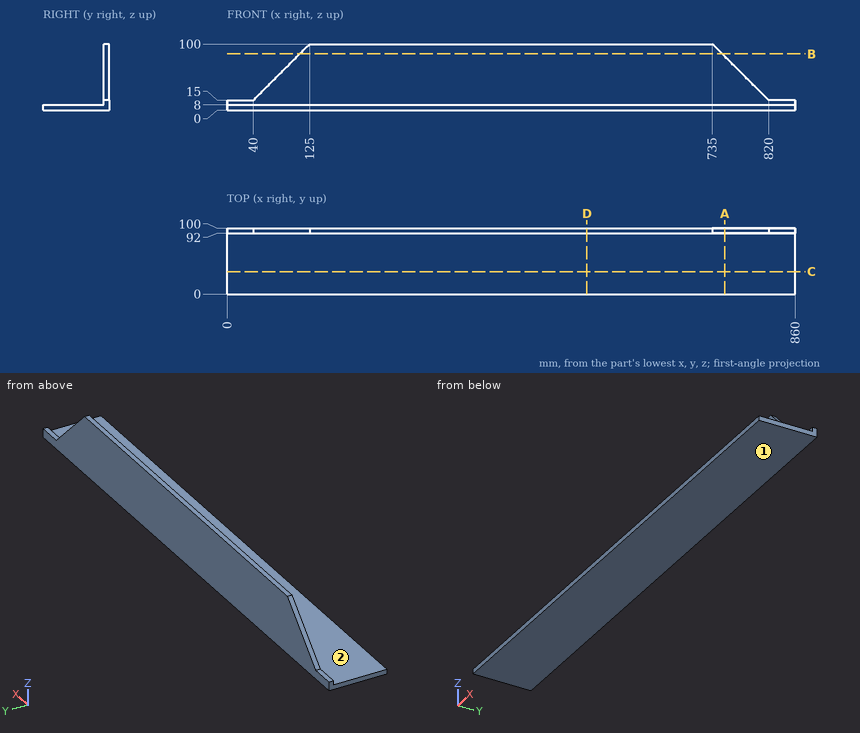
The figure shows three views and two pictorial views of one solid part (mm, origin at its lowest corner). Answer the questions. A direction names the side the tool comes from. Give positions to 0.01 mm unless a question says otherwise; leave off trailing zeros. Order: outer loops, then holes, each group sorted by start corner. A loop starts at its lowest first (then second) coordinate and runs counter-clockwise, first axis right, second up. Notation, with made-up numbers: (-14, 23.5) -> (-7, 23.5) arc R31 ccw to (-7, 58.5) -> close; hole circle Ø4 at (4, 11). An arc over 180 degrees is marked (long way). Answer as CSV lines item,"result". Start each with the question number.
(1) Section C-C, the plane y = 34 is taken. Write down the section's boundary in (x, z), plus the area to 3 significant figures.
(2) Section D-D, the plane x = 545 is taken. Write down the section's boundary in (y, z).
(3) Consider line 1 along Z through (x, y) = (419, 37); line 2 along Y through (x, z) = (596.5, 57); line 3 along X through (y, z) = (96, 79). Determine where each line is inside the solid, lowest interval first.
(4) Each of these flat-tipped pins is pushed along its axis until it touches: pin 1 Ø5 at (x, y) = (581.5, 38) entering from +Z; pin 2 Ø2.5 at (x, y) = (847, 95) entering from +Z; pin 3 Ø10 at (x, y) = (380, 82) entering from -Z. Where does it stop, or does it pass through?
(5) Section B-B, the plane z = 85 is taken. Write down the section's boundary in (x, y), plus the area to 3 significant figures.
(6) Section A-A, the plane x = 754 is taken. Write down the section's boundary in (y, z).
(7) Which of the six approach directions +Z, -Z, +X, -X, +Y, -Y give full straight-line access (tool end or side, diameter ignored) to the marked faces 1 and 2?
Entries:
1,outline,"(0, 0) -> (860, 0) -> (860, 8) -> (0, 8) -> close"
1,area,"6,880 mm²"
2,outline,"(0, 0) -> (100, 0) -> (100, 100) -> (92, 100) -> (92, 8) -> (0, 8) -> close"
3,line 1,"0 to 8"
3,line 2,"92 to 100"
3,line 3,"104 to 756"
4,pin 1,"z = 8"
4,pin 2,"z = 15"
4,pin 3,"z = 0"
5,outline,"(110, 92) -> (750, 92) -> (750, 100) -> (110, 100) -> close"
5,area,"5,120 mm²"
6,outline,"(0, 0) -> (100, 0) -> (100, 81) -> (92, 81) -> (92, 8) -> (0, 8) -> close"
7,face 1,"-Z, +X, -X, +Y, -Y"
7,face 2,"+Z, +X, -X, -Y"
